from build123d import *

# Parameters (mm, degrees)
SKETCH_2_W               = 30
SKETCH_2_H               = 30
EXTRUDE_1_DEPTH          = 225
SKETCH_4_W               = 26
SKETCH_4_H               = 26
CUT_EXTRUDE_1_DEPTH      = 226
CUT_EXTRUDE_1_DEPTH_BACK = 226
SKETCH_5_R               = 2.025
CUT_EXTRUDE_2_DEPTH      = 1
CUT_EXTRUDE_2_DEPTH_BACK = 31
SKETCH_7_R               = 1.525
CUT_EXTRUDE_3_DEPTH      = 1
CUT_EXTRUDE_3_DEPTH_BACK = 31
SKETCH_8_R               = 1.525
CUT_EXTRUDE_4_DEPTH      = 31
PATTERN_LINEAR_1_COUNT   = 13
PATTERN_LINEAR_1_PITCH   = 30
SKETCH_9_R               = 3.8
CUT_EXTRUDE_5_DEPTH      = 5
CUT_EXTRUDE_6_DEPTH      = 5
PATTERN_LINEAR_2_COUNT   = 7
PATTERN_LINEAR_2_PITCH   = 57
SKETCH_11_R              = 2.025
CUT_EXTRUDE_7_DEPTH      = 1
CUT_EXTRUDE_7_DEPTH_BACK = 31
CUT_EXTRUDE_8_DEPTH      = 10
SKETCH_14_R              = 1.525
CUT_EXTRUDE_9_DEPTH      = 1
CUT_EXTRUDE_9_DEPTH_BACK = 31
SKETCH_15_R              = 7.5
CUT_EXTRUDE_10_DEPTH     = 2


with BuildPart() as part:
    # 草图2 → 凸台-拉伸1 (new body, symmetric)
    with BuildSketch(Plane(origin=(0, 0, 0), x_dir=(1, 0, 0), z_dir=(0, 1, 0))):
        Rectangle(SKETCH_2_W, SKETCH_2_H)
    extrude(amount=EXTRUDE_1_DEPTH, both=True)

    # 草图4 → 切除-拉伸1 (cut, two sides)
    with BuildSketch(Plane(origin=(0, 0, 0), x_dir=(1, 0, 0), z_dir=(0, 1, 0))) as cut_extrude_1_sk:
        Rectangle(SKETCH_4_W, SKETCH_4_H)
    extrude(amount=CUT_EXTRUDE_1_DEPTH, mode=Mode.SUBTRACT)
    extrude(cut_extrude_1_sk.sketch, amount=-CUT_EXTRUDE_1_DEPTH_BACK, mode=Mode.SUBTRACT)

    # 草图5 → 切除-拉伸2 (cut, two sides)
    with BuildSketch(Plane(origin=(0, 0, -15), x_dir=(-1, 0, 0), z_dir=(0, 0, -1))) as cut_extrude_2_sk:
        with Locations((-7.5, 210)):
            Circle(SKETCH_5_R)
        with Locations((7.5, 210)):
            Circle(SKETCH_5_R)
        with Locations((-7.5, 195)):
            Circle(SKETCH_5_R)
        with Locations((7.5, 195)):
            Circle(SKETCH_5_R)
    extrude(amount=CUT_EXTRUDE_2_DEPTH, mode=Mode.SUBTRACT)
    extrude(cut_extrude_2_sk.sketch, amount=-CUT_EXTRUDE_2_DEPTH_BACK, mode=Mode.SUBTRACT)

    # 草图7 → 切除-拉伸3 (cut, two sides)
    with BuildSketch(Plane(origin=(15, 0, 0), x_dir=(0, 0, -1), z_dir=(1, 0, 0))) as cut_extrude_3_sk:
        with Locations((-6.5, 202.499999999)):
            Circle(SKETCH_7_R)
        with Locations((6.5, 202.499999999)):
            Circle(SKETCH_7_R)
    extrude(amount=CUT_EXTRUDE_3_DEPTH, mode=Mode.SUBTRACT)
    extrude(cut_extrude_3_sk.sketch, amount=-CUT_EXTRUDE_3_DEPTH_BACK, mode=Mode.SUBTRACT)

    # 草图8 → 切除-拉伸4 (cut, through all)
    with BuildSketch(Plane.ZY.offset(15)):
        with Locations((0, -170.000000001)):
            Circle(SKETCH_8_R)
    cut_extrude_4 = extrude(amount=-CUT_EXTRUDE_4_DEPTH, mode=Mode.SUBTRACT)

    # 阵列(线性)1: 切除-拉伸4 ×13
    with Locations(*[(0, i * PATTERN_LINEAR_1_PITCH, 0) for i in range(1, PATTERN_LINEAR_1_COUNT)]):
        add(cut_extrude_4, mode=Mode.SUBTRACT)

    # 草图9 → 切除-拉伸5 (cut)
    with BuildSketch(Plane(origin=(0, 0, -15), x_dir=(-1, 0, 0), z_dir=(0, 0, -1))):
        with Locations((-7.5, 210)):
            Circle(SKETCH_9_R)
        with Locations((7.5, 210)):
            Circle(SKETCH_9_R)
        with Locations((7.5, 195)):
            Circle(SKETCH_9_R)
        with Locations((-7.5, 195)):
            Circle(SKETCH_9_R)
    extrude(amount=-CUT_EXTRUDE_5_DEPTH, mode=Mode.SUBTRACT)

    # 草图10 → 切除-拉伸6 (cut)
    with BuildSketch(Plane(origin=(0, 0, -15), x_dir=(-1, 0, 0), z_dir=(0, 0, -1))):
        with BuildLine():
            Line((-9, -196.5), (-9, -165.5))
            ThreePointArc((-9, -165.5), (0, -156.5), (9, -165.5))
            Line((9, -165.5), (9, -196.5))
            ThreePointArc((9, -196.5), (0, -205.5), (-9, -196.5))
        make_face()
    cut_extrude_6 = extrude(amount=-CUT_EXTRUDE_6_DEPTH, mode=Mode.SUBTRACT)

    # 阵列(线性)2: 切除-拉伸6 ×7
    with Locations(*[(0, i * PATTERN_LINEAR_2_PITCH, 0) for i in range(1, PATTERN_LINEAR_2_COUNT)]):
        add(cut_extrude_6, mode=Mode.SUBTRACT)

    # 草图11 → 切除-拉伸7 (cut, two sides)
    with BuildSketch(Plane.ZY.offset(15)) as cut_extrude_7_sk:
        with Locations((-9, -187)):
            Circle(SKETCH_11_R)
        with Locations((9, -187)):
            Circle(SKETCH_11_R)
        with Locations((-9, -217)):
            Circle(SKETCH_11_R)
        with Locations((9, -217)):
            Circle(SKETCH_11_R)
    extrude(amount=CUT_EXTRUDE_7_DEPTH, mode=Mode.SUBTRACT)
    extrude(cut_extrude_7_sk.sketch, amount=-CUT_EXTRUDE_7_DEPTH_BACK, mode=Mode.SUBTRACT)

    # 草图13 → 切除-拉伸8 (cut)
    with BuildSketch(Plane.XY.offset(15)):
        with BuildLine():
            Line((-6, 190), (6, 190))
            ThreePointArc((6, 190), (8.121320344, 189.121320344), (9, 187))
            Line((9, 187), (9, 173))
            ThreePointArc((9, 173), (8.121320344, 170.878679656), (6, 170))
            Line((6, 170), (-6, 170))
            ThreePointArc((-6, 170), (-8.121320344, 170.878679656), (-9, 173))
            Line((-9, 173), (-9, 187))
            ThreePointArc((-9, 187), (-8.121320344, 189.121320344), (-6, 190))
        make_face()
        with BuildLine():
            Line((9, 135), (9, 125))
            ThreePointArc((9, 125), (0, 116), (-9, 125))
            Line((-9, 125), (-9, 135))
            ThreePointArc((-9, 135), (0, 144), (9, 135))
        make_face()
        with BuildLine():
            Line((-9, 65), (-9, 75))
            ThreePointArc((-9, 75), (0, 84), (9, 75))
            Line((9, 75), (9, 65))
            ThreePointArc((9, 65), (0, 56), (-9, 65))
        make_face()
        with BuildLine():
            Line((-9, 5), (-9, 15))
            ThreePointArc((-9, 15), (0, 24), (9, 15))
            Line((9, 15), (9, 5))
            ThreePointArc((9, 5), (0, -4), (-9, 5))
        make_face()
    extrude(amount=-CUT_EXTRUDE_8_DEPTH, mode=Mode.SUBTRACT)

    # 草图14 → 切除-拉伸9 (cut, two sides)
    with BuildSketch(Plane(origin=(0, 0, -15), x_dir=(-1, 0, 0), z_dir=(0, 0, -1))) as cut_extrude_9_sk:
        with Locations((-0.05, 202.5)):
            Circle(SKETCH_14_R)
    extrude(amount=CUT_EXTRUDE_9_DEPTH, mode=Mode.SUBTRACT)
    extrude(cut_extrude_9_sk.sketch, amount=-CUT_EXTRUDE_9_DEPTH_BACK, mode=Mode.SUBTRACT)

    # 草图15 → 切除-拉伸10 (cut)
    with BuildSketch(Plane(origin=(0, 0, 13), x_dir=(-1, 0, 0), z_dir=(0, 0, -1))):
        with Locations((0, -200)):
            Circle(SKETCH_15_R)
    extrude(amount=-CUT_EXTRUDE_10_DEPTH, mode=Mode.SUBTRACT)


solid = part.part
Geometry check sheet. Reference: the model listing, model coordinates, mm. A direction names the side the tool comes from. Round coordinates to 2 decimals unless told otherwise and drop trailing zeros. Order: outer loops, then holes, each group sorted by start corner. A loop starts at its lowest first (then second) coordinate and runs counter-clockwise, first axis right, second up. Notation, with made-up numbers: (23, -39) -> (76, -39) arc R14 cw to (76, -24) -> close; hole circle Ø9 at (38, 49). An arc over 180 degrees is marked (long way). Use one line per item in the form item = value.
1. Cross-section at A-A, the plane y = -65. Enter the section's corners in (x, z).
Working result:
outline = (-15, -15) -> (-9, -15) -> (-9, -13) -> (-13, -13) -> (-13, 13) -> (13, 13) -> (13, -13) -> (9, -13) -> (9, -15) -> (15, -15) -> (15, 15) -> (-15, 15) -> close
2. Mould release check, pull along Y, two halves, no side actions. Record for faces 1 (the face through (-0.198, -34.498, -14.014)), 2 (the face through (0, 144, 14)), 3 (the face through (-12, 3, -13)): pulls with the +Y half, pulls with the -Y half, needs draft (parallel to the pull), parting line crosses it, or undercut.
Working result:
face_1 = undercut
face_2 = undercut
face_3 = needs draft
3. Set-up check for faces 4 (the face through (13, 3, 0)), 5 (the face through (0.198, 128.498, -14.014)), 6 (the face through (0, 116, 14)), 7 (the face through (0, -4, 14)): record each of +Z, -Z, +X, -X, +Y, -Y from which the full face is reachable in a straight line by a thin tool's end or side.
Working result:
face_4 = +Y, -Y
face_5 = -Z
face_6 = +Z
face_7 = +Z, -Z
4. Go/stop test with a flat-tipped pin: pin 1 (4.5 mm diameter, centred on x = -7.5, y = 210, fed in from -Z). Record where the tip stops, or that it passes through.
Working result:
pin_1 = 13
5. Scan lines: line 1 along Z through (x, y) = (-13.9, -187) (3 decimals); line 2 along Y through (x, z) = (-13.8, -9) (3 decimals); line 3 along X through (y, z) = (120, -12.5). Record each from-to range of solid material in increasing order. Write a range as from..to.
Working result:
line_1 = -15..-11.025, -6.975..6.975, 11.025..15
line_2 = -225..-219.025, -214.975..-189.025, -184.975..225
line_3 = -15..-13, 13..15
